For this review, use the dimensioned drawing (mm, ordinates from the lowest corner) and the shaded views. Give positions to 0.01 mm unless a question says otherwise; leave off trailing zeros. Write each loop counter-clockwise with the first axis right and the second up, starting at its lowest first coordinate (ties: lowest second). Pieces come first, ordered by that corner, then holes. Notation, with made-up numbers: (14, 13) - (30, 13) arc R13 cw to (30, 32) - close; hole circle Ø11 at (-26.75, 10.25). An arc over 180 degrees is marked (long way). One line per question, with ' | ' between items. Start each with the question number.
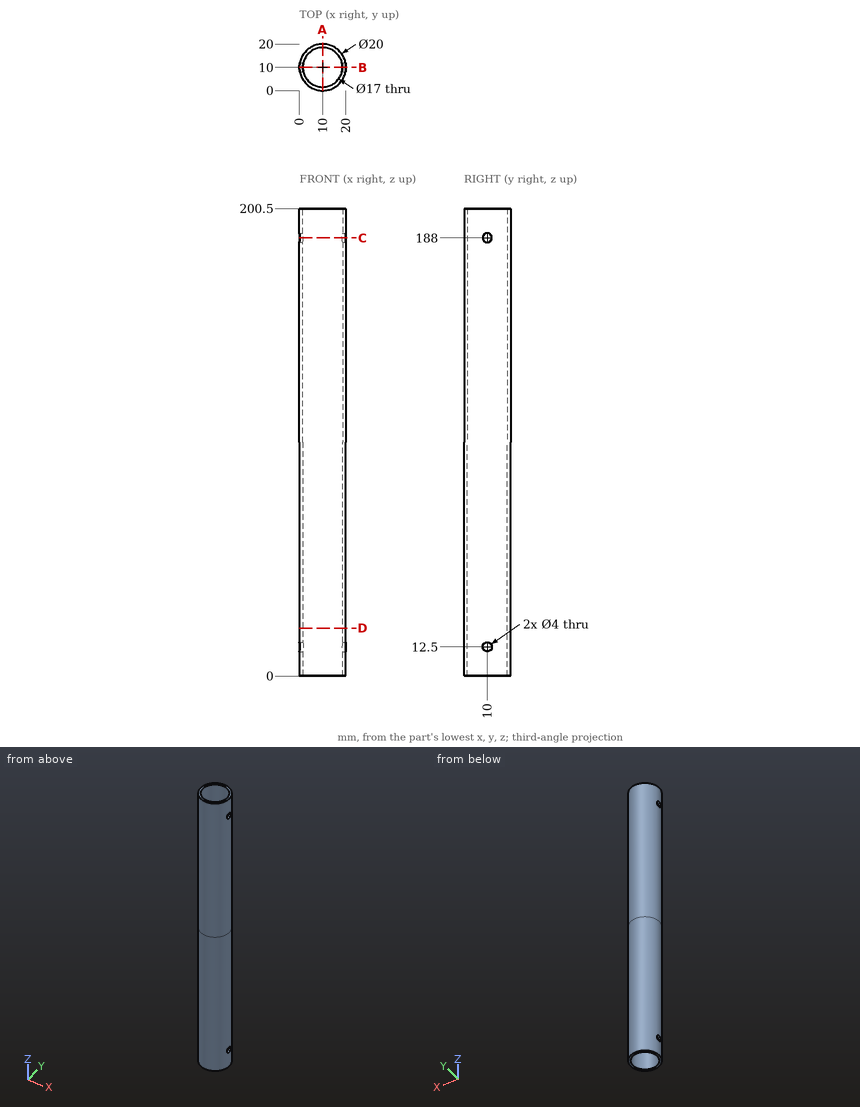
Item 1: Take a section at A-A (x = 10). Give the boundary of the cut face in (y, z), plus the area to 4 significant figures.
Item 2: Take a section at D-D (z = 20.5). Give the boundary of the cut face in (x, y), plus the area to 3 significant figures.
Item 3: For probe 1 along Y at (x, z) = (10, 63); probe 2 along X at (y, z) = (13, 88); probe 3 along Y at (x, z) = (3.5, 110.5), list the stretches that pass through material, from the lowest coordinate up.
Item 4: Clearance check with flat-ended pins moving along their axes: P1, Ø5, axis at y = 17.5, z = 54.5, coming from the +X side; P2, Ø6, axis at x = 15.5, z = 55, coming from the +Y side; P3, Ø8, axis at x = 5, z = 99, coming from the -Y side; P4, Ø6.5, axis at y = 10, z = 12.5, coming from the -X side. State where each tip first meets the part, or that it passes through.
Item 5: Take a section at C-C (z = 188). Give the boundary of the cut face in (x, y).
Item 6: Take a section at B-B (y = 10). Give the boundary of the cut face in (x, z), plus the area to 4 significant figures.
Check sheet entries:
1) outline: (0, 0) - (1.5, 0) - (1.5, 200.5) - (0, 200.5) - close; (18.5, 0) - (20, 0) - (20, 200.5) - (18.5, 200.5) - close | area: 601.5 mm^2
2) outline: circle Ø20 at (10, 10); hole circle Ø17 at (10, 10) | area: 87.2 mm^2
3) probe 1: y = 0 to 1.5, 18.5 to 20 | probe 2: x = 0.46 to 2.05, 17.95 to 19.54 | probe 3: y = 2.4 to 4.52, 15.48 to 17.6
4) P1: stops at x = 18.66 | P2: stops at y = 19.68 | P3: stops at y = 0.05 | P4: stops at x = 0
5) outline: (0.2, 8) arc R10 ccw to (19.8, 8) - (18.26, 8) arc R8.5 cw to (1.74, 8) - close; (0.2, 12) - (1.74, 12) arc R8.5 cw to (18.26, 12) - (19.8, 12) arc R10 ccw to start
6) outline: (0, 0) - (1.5, 0) - (1.5, 10.5) - (0, 10.5) - close; (0, 14.5) - (1.5, 14.5) - (1.5, 186) - (0, 186) - close; (0, 190) - (1.5, 190) - (1.5, 200.5) - (0, 200.5) - close; (18.5, 0) - (20, 0) - (20, 10.5) - (18.5, 10.5) - close; (18.5, 14.5) - (20, 14.5) - (20, 186) - (18.5, 186) - close; (18.5, 190) - (20, 190) - (20, 200.5) - (18.5, 200.5) - close | area: 577.5 mm^2
